Verification items for the finished model (mm, model axes). A direction names the side the tool comes from. Round coordinates to 2 decimals unless told otherwise and drop trailing zeros. Write each loop counter-clockwise with the first axis right and the second up, starting at its lowest first coordinate (ties: lowest second). Pieces come first, ordered by that corner, then holes. Notation, with made-up numbers: (65, 32.25) - (114, 32.25) arc R14 cw to (114, 37.25) - close; hole circle Ø10 at (78, -10.75). An arc over 180 degrees is marked (long way). Answer as a JSON object with one key per item and string values. Group by question number.
1) Go/stop test with flat-tipped pins: pin 1 Ø16 at (x, y) = (-105, 8.5) entering from -Z; pin 2 Ø3 at (x, z) = (74.5, -56) entering from +Y; pin 3 Ø6 at (x, z) = (144, -58.5) entering from +Y. Record where each tip stops, or that it passes through.
2) Thickness scan on line 1 (X direction, y = 1.5, z = 67); line 2 (X direction, y = 6.5, z = 65.5); line 3 (Y direction, x = 55.5, z = -63.5). Record the ranges inside material, lowest first.
3) Section check B-B (x = -101.5). Enter the section's corners in (y, z), then the cut area to 3 significant figures.
4) Section check C-C (x = -135.5). Enter the section's corners in (y, z), then the cut area to 3 significant figures.
5) Mould release check, pull along Y, two halves, no side actions. Record for faces 1 (the flat face through (-100, 0, 65)), 2 (the flat face through (-130, 14, -65)), 3 (the flat face through (140, 7, -65)), 4 (the flat face through (-60, 7, 65)): +Y half, -Y half, draft (parallel to the pull), parting line (faces both ways), or undercut.
6) Set-up check for faces 5 (the flat face through (70, 14, 65)), 6 (the flat face through (70, 14, -65)), 7 (the flat face through (-140, 7, 65)), 8 (the flat face through (-140, 7, -65)): record each of +Z, -Z, +X, -X, +Y, -Y from which the full face is reachable in a straight line by a thin tool's end or side.
```python
from build123d import *

# Parameters (mm, degrees)
SKETCH1_W               = 320
SKETCH1_H               = 160
BOSS_EXTRUDE1_DEPTH     = 20
SKETCH2_W               = 60
SKETCH2_H               = 30
CUT_EXTRUDE1_DEPTH      = 28
SKETCH3_W               = 20
SKETCH3_H               = 5
CUT_EXTRUDE3_DEPTH      = 30
MIRROR3_COPY_1_SKETCH_W = 60
MIRROR3_COPY_1_SKETCH_H = 30
MIRROR3_COPY_1_DEPTH    = 28
MIRROR3_COPY_2_SKETCH_W = 20
MIRROR3_COPY_2_SKETCH_H = 5
MIRROR3_COPY_2_DEPTH    = 30
SKETCH8_W               = 18
SKETCH8_H               = 9
CUT_EXTRUDE6_DEPTH      = 30
SKETCH9_W               = 18
SKETCH9_H               = 9
CUT_EXTRUDE7_DEPTH      = 30
SKETCH10_W              = 320
SKETCH10_H              = 160
BOSS_EXTRUDE2_DEPTH     = 10


with BuildPart() as part:
    # Sketch1 → Boss-Extrude1 (new body)
    with BuildSketch(Plane(origin=(0, 0, 0), x_dir=(1, 0, 0), z_dir=(0, 1, 0))):
        Rectangle(SKETCH1_W, SKETCH1_H)
    extrude(amount=BOSS_EXTRUDE1_DEPTH)

    # Sketch2 → Cut-Extrude1 (cut)
    with BuildSketch(Plane(origin=(0, 20, 0), x_dir=(1, 0, 0), z_dir=(0, 1, 0))):
        with Locations((-100, -65)):
            Rectangle(SKETCH2_W, SKETCH2_H)
    cut_extrude1 = extrude(amount=-CUT_EXTRUDE1_DEPTH, mode=Mode.SUBTRACT)

    # Sketch3 → Cut-Extrude3 (cut)
    with BuildSketch(Plane.XY.offset(80)):
        with Locations((-140, 4.5)):
            Rectangle(SKETCH3_W, SKETCH3_H)
        with Locations((-60, 4.5)):
            Rectangle(SKETCH3_W, SKETCH3_H)
    cut_extrude3 = extrude(amount=-CUT_EXTRUDE3_DEPTH, mode=Mode.SUBTRACT)

    # Mirror2: Cut-Extrude1, Cut-Extrude3 across plane
    add(cut_extrude1.mirror(Plane(origin=(0, 0, 0), x_dir=(0, 0, 1), z_dir=(1, 0, 0))), mode=Mode.SUBTRACT)
    add(cut_extrude3.mirror(Plane(origin=(0, 0, 0), x_dir=(0, 0, 1), z_dir=(1, 0, 0))), mode=Mode.SUBTRACT)

    # Mirror3: Cut-Extrude1, Cut-Extrude3 across plane
    add(cut_extrude1.mirror(Plane.XY), mode=Mode.SUBTRACT)
    add(cut_extrude3.mirror(Plane.XY), mode=Mode.SUBTRACT)

    # Mirror3 copy 1 sketch → Mirror3 copy 1 (cut)
    with BuildSketch(Plane(origin=(0, 20, 0), x_dir=(-1, 0, 0), z_dir=(0, 1, 0))):
        with Locations((-100, -65)):
            Rectangle(MIRROR3_COPY_1_SKETCH_W, MIRROR3_COPY_1_SKETCH_H)
    extrude(amount=-MIRROR3_COPY_1_DEPTH, mode=Mode.SUBTRACT)

    # Mirror3 copy 2 sketch → Mirror3 copy 2 (cut)
    with BuildSketch(Plane(origin=(0, 0, -80), x_dir=(-1, 0, 0), z_dir=(0, 0, -1))):
        with Locations((-140, 4.5)):
            Rectangle(MIRROR3_COPY_2_SKETCH_W, MIRROR3_COPY_2_SKETCH_H)
        with Locations((-60, 4.5)):
            Rectangle(MIRROR3_COPY_2_SKETCH_W, MIRROR3_COPY_2_SKETCH_H)
    extrude(amount=-MIRROR3_COPY_2_DEPTH, mode=Mode.SUBTRACT)

    # Sketch8 → Cut-Extrude6 (cut)
    with BuildSketch(Plane(origin=(0, 0, -80), x_dir=(-1, 0, 0), z_dir=(0, 0, -1))):
        with Locations((-139, 15.5)):
            Rectangle(SKETCH8_W, SKETCH8_H)
    cut_extrude6 = extrude(amount=-CUT_EXTRUDE6_DEPTH, mode=Mode.SUBTRACT)

    # Sketch9 → Cut-Extrude7 (cut)
    with BuildSketch(Plane(origin=(0, 0, -80), x_dir=(-1, 0, 0), z_dir=(0, 0, -1))):
        with Locations((61, 15.5)):
            Rectangle(SKETCH9_W, SKETCH9_H)
    cut_extrude7 = extrude(amount=-CUT_EXTRUDE7_DEPTH, mode=Mode.SUBTRACT)

    # Sketch10 → Boss-Extrude2 (add)
    with BuildSketch(Plane.XZ):
        Rectangle(SKETCH10_W, SKETCH10_H)
    extrude(amount=BOSS_EXTRUDE2_DEPTH)

    # Mirror4: Cut-Extrude6, Cut-Extrude7 across plane
    add(cut_extrude6.mirror(Plane.XY), mode=Mode.SUBTRACT)
    add(cut_extrude7.mirror(Plane.XY), mode=Mode.SUBTRACT)


solid = part.part
```
Returned:
{
 "1": {"pin 1": "z = -50", "pin 2": "y = 0", "pin 3": "y = 11"},
 "2": {"line 1": "-160 to -130, -70 to 70, 130 to 160", "line 2": "-160 to -150, -50 to 50, 150 to 160", "line 3": "-10 to 2, 7 to 20"},
 "3": {"outline": "(-10, -80) - (0, -80) - (0, -50) - (20, -50) - (20, 50) - (0, 50) - (0, 80) - (-10, 80) - close", "area": "3,600 mm2"},
 "4": {"outline": "(-10, -80) - (2, -80) - (2, -50) - (7, -50) - (7, -80) - (20, -80) - (20, 80) - (7, 80) - (7, 50) - (2, 50) - (2, 80) - (-10, 80) - close", "area": "4,500 mm2"},
 "5": {"face 1": "+Y half", "face 2": "draft", "face 3": "undercut", "face 4": "undercut"},
 "6": {"face 5": "+Z, +Y", "face 6": "-Z, +Y", "face 7": "+Z", "face 8": "-Z"}
}
